Autodesk Inventor part; units mm, degrees
ref_plane "YZ Plane" through (0, 0, 0) normal (1, 0, 0) x (0, 1, 0)
ref_plane "XZ Plane" through (0, 0, 0) normal (0, 1, 0) x (-1, 0, 0)
ref_plane "XY Plane" through (0, 0, 0) normal (0, 0, 1) x (1, 0, 0)
sketch "Sketch1" plane through (0, 0, 0) normal (0, 1, 0) x (-1, 0, 0)
  line L0 (0, 0) -> (20, 0)
  line L1 (20, 0) -> (20, -20)
  line L2 (20, -20) -> (0, -20)
  line L3 (0, -20) -> (0, 0)
  dimension "d0" = 20
  dimension "d1" = 20
extrude "Extrusion1" add sketch "Sketch1" along normal blind 2
sketch "Sketch2" plane through (0, 2, 0) normal (0, 1, 0) x (1, 0, 0)
  line L0 (0, 20) -> (-20, 20)
  line L1 (-20, 20) -> (-20, 0)
  line L2 (-20, 0) -> (0, 0)
  line L3 (0, 0) -> (0, 20)
  line L4 (-18, 2) -> (-18, 18)
  line L5 (-18, 18) -> (-2, 18)
  line L6 (-2, 18) -> (-2, 2)
  line L7 (-2, 2) -> (-18, 2)
  line L8 (-16.75, 16.75) -> (-16.75, 3.25)
  line L9 (-16.75, 3.25) -> (-3.25, 3.25)
  line L10 (-3.25, 3.25) -> (-3.25, 16.75)
  line L11 (-3.25, 16.75) -> (-16.75, 16.75)
  dimension "d4" = 2
  dimension "d5" = 1.25
extrude "Extrusion2" add sketch "Sketch2" along normal blind 2 contours L4 L5 L6 L7
extrude "Extrusion3" cut sketch "Sketch2" against normal blind 10 contours L11 L10 L9 L8
sketch "Sketch3" plane through (0, 0, 0) normal (0, -1, 0) x (1, 0, 0)
  line L0 (-3.25, -3.25) -> (-3.25, -16.75)
  line L1 (-3.25, -16.75) -> (-16.75, -16.75)
  line L2 (-16.75, -16.75) -> (-16.75, -3.25)
  line L3 (-16.75, -3.25) -> (-3.25, -3.25)
  line L4 (0, -20) -> (-20, -20)
  line L5 (0, 0) -> (0, -20)
  line L6 (-20, 0) -> (0, 0)
  line L7 (-20, -20) -> (-20, 0)
  line L8 (-6, -6) -> (-6, -14)
  line L9 (-6, -14) -> (-14, -14)
  line L10 (-14, -14) -> (-14, -6)
  line L11 (-14, -6) -> (-6, -6)
extrude "Extrusion4" add sketch "Sketch3" against normal up to surface (2 mm away) contours L0 L1 L2 L3
extrude "Extrusion5" add sketch "Sketch3" against normal blind 11.5 contours L8 L9 L10 L11
move faces "Move1" translate (0, 3, 0) faces at (-11.3333, 11.5, -8.6667)
properties part number "latticeChamberCapv4"
Geometry check sheet. Reference: the model listing, model coordinates, mm. A direction names the side the tool comes from. Give positions to 0.01 mm unless a question says otherwise; leave off trailing zeros. Order: outer loops, then holes, each group sorted by start corner. A loop starts at its lowest first (then second) coordinate and runs counter-clockwise, first axis right, second up.
1. Release check for a two-part mould opening along X. For faces 1 (the face through (-10, 3, -16.75)), 2 (the face through (-20, 1, -10)), 3 (the face through (-10, 1, 0)), 4 (the face through (0, 1, -10)) record: pulls with the +X half, pulls with the -X half, needs draft (parallel to the pull), parting line crosses it, or undercut.
2. Section check A-A, the plane y = 3. Enter the section's corners in (x, z).
3. Access from +Z, -Z, +X, -X, +Y, -Y to the whole of each face (thin tool, end or side, straight path). Record for faces 5 (the face through (-10, 3, -3.25)), 6 (the face through (-10, 3, -18)), 7 (the face through (-10, 3, -2)).
4. Thickness scan on L1, parallel to Y at x = -11.5, z = -5.25; L2, parallel to Y at x = -2.25, z = -15.25; L3, parallel to Z at x = -13, y = 6.5. Record the ranges inside material, lowest first.
5. Section check B-B, the plane x = -8.5. Enter the section's corners in (y, z), and give its area (3 significant figures).
6. Section check C-C, the plane z = -8. Enter the section's corners in (x, y), and give its area (3 significant figures).
7. Section check D-D, the plane y = 9.25. Enter the section's corners in (x, z), and give its area (3 significant figures).
8. Gauge pin test, flat ends, axial feed: pin 1 Ø1 at (x, y) = (-13, 3) entering from -Z; pin 2 Ø1.6 at (x, y) = (-10.5, 3) entering from +Z; pin 3 Ø4 at (x, z) = (-17, -13) entering from +Y. Record the tip position at first contact, or that the pin passes through.
Values follow:
1. face 1: undercut
1. face 2: pulls with the -X half
1. face 3: needs draft
1. face 4: pulls with the +X half
2. outline: (-18, -18) - (-2, -18) - (-2, -2) - (-18, -2) - close; (-14, -14) - (-6, -14) - (-6, -6) - (-14, -6) - close; hole (-16.75, -16.75) - (-3.25, -16.75) - (-3.25, -3.25) - (-16.75, -3.25) - close
3. face 5: +Y
3. face 6: -Z, +X, -X, +Y
3. face 7: +Z, +X, -X, +Y
4. L1: y = 0 to 2
4. L2: y = 0 to 4
4. L3: z = -14 to -6
5. outline: (0, -20) - (2, -20) - (2, -18) - (4, -18) - (4, -16.75) - (2, -16.75) - (2, -14) - (14.5, -14) - (14.5, -6) - (2, -6) - (2, -3.25) - (4, -3.25) - (4, -2) - (2, -2) - (2, 0) - (0, 0) - close
5. area: 145 mm2
6. outline: (-20, 0) - (0, 0) - (0, 2) - (-2, 2) - (-2, 4) - (-3.25, 4) - (-3.25, 2) - (-6, 2) - (-6, 14.5) - (-14, 14.5) - (-14, 2) - (-16.75, 2) - (-16.75, 4) - (-18, 4) - (-18, 2) - (-20, 2) - close
6. area: 145 mm2
7. outline: (-14, -14) - (-6, -14) - (-6, -6) - (-14, -6) - close
7. area: 64.0 mm2
8. pin 1: stops at z = -18
8. pin 2: stops at z = -2
8. pin 3: stops at y = 4
